Geometry: final body of the model. Coordinates: model frame, mm. A direction names the side the tool comes from. Give positions to 0.01 mm unless a question says otherwise; leave off trailing zeros. Order: outer loops, then holes, each group sorted by start corner. A loop starts at its lowest first (then second) coordinate and runs counter-clockwise, first axis right, second up. Notation, with made-up numbers: (10.5, -1.75) -> (61.5, -1.75) arc R12 cw to (61.5, 13.25) -> close; hole circle Ø3 at (55, 54.5). An arc over 180 degrees is marked (long way). One line per question, with ' | ' between items.
from build123d import *

# Parameters (mm, degrees)
SKETCH1_R           = 30
BOSS_EXTRUDE1_DEPTH = 4
BOSS_EXTRUDE2_START = -17
BOSS_EXTRUDE2_DEPTH = 17


with BuildPart() as part:
    # Sketch1 → Boss-Extrude1 (new body)
    with BuildSketch(Plane.XY):
        Circle(SKETCH1_R)
        with BuildLine():
            ThreePointArc((-12.727922061, -12.727922061), (0, -18), (12.727922061, -12.727922061))
            ThreePointArc((12.727922061, -12.727922061), (13.378240315, -9.458551421), (10.606601718, -7.606601718))
            ThreePointArc((10.606601718, -7.606601718), (9.458551421, -7.83496312), (8.485281374, -8.485281374))
            ThreePointArc((8.485281374, -8.485281374), (0, -12), (-8.485281374, -8.485281374))
            ThreePointArc((-8.485281374, -8.485281374), (-9.458551421, -7.83496312), (-10.606601718, -7.606601718))
            ThreePointArc((-10.606601718, -7.606601718), (-13.378240315, -9.458551421), (-12.727922061, -12.727922061))
        make_face(mode=Mode.SUBTRACT)
        with BuildLine():
            ThreePointArc((8.485281374, 8.485281374), (12.727922061, 8.485281374), (12.727922061, 12.727922061))
            ThreePointArc((12.727922061, 12.727922061), (6.888301783, 16.629831585), (0, 18))
            ThreePointArc((0, 18), (-6.888301783, 16.629831585), (-12.727922061, 12.727922061))
            ThreePointArc((-12.727922061, 12.727922061), (-12.727922061, 8.485281374), (-8.485281374, 8.485281374))
            ThreePointArc((-8.485281374, 8.485281374), (-4.592201188, 11.08655439), (0, 12))
            ThreePointArc((0, 12), (4.592201188, 11.08655439), (8.485281374, 8.485281374))
        make_face(mode=Mode.SUBTRACT)
        with BuildLine():
            ThreePointArc((0, -4.95), (-1.55, -6.5), (0, -8.05))
            ThreePointArc((0, -8.05), (1.55, -6.5), (0, -4.95))
        make_face(mode=Mode.SUBTRACT)
        with BuildLine():
            ThreePointArc((6, 1.55), (4.45, 0), (6, -1.55))
            ThreePointArc((6, -1.55), (7.55, 0), (6, 1.55))
        make_face(mode=Mode.SUBTRACT)
        with BuildLine():
            ThreePointArc((-6, 1.55), (-7.55, 0), (-6, -1.55))
            ThreePointArc((-6, -1.55), (-4.45, 0), (-6, 1.55))
        make_face(mode=Mode.SUBTRACT)
        with BuildLine():
            ThreePointArc((0, 4.95), (1.55, 6.5), (0, 8.05))
            ThreePointArc((0, 8.05), (-1.55, 6.5), (0, 4.95))
        make_face(mode=Mode.SUBTRACT)
        with BuildLine():
            ThreePointArc((0, 4.1), (-4.1, 0), (0, -4.1))
            ThreePointArc((0, -4.1), (4.1, 0), (0, 4.1))
        make_face(mode=Mode.SUBTRACT)
    extrude(amount=-BOSS_EXTRUDE1_DEPTH)

    # Sketch2 → Boss-Extrude2 (add)
    with BuildSketch(Plane(origin=(0, 0, -21), x_dir=(-1, 0, 0), z_dir=(0, 0, -1)).offset(BOSS_EXTRUDE2_START)):
        with BuildLine():
            ThreePointArc((0, -30), (30, 0), (0, 30))
            ThreePointArc((0, 30), (-30, 0), (0, -30))
        make_face()
        with BuildLine():
            ThreePointArc((0, 21), (-21, 0), (0, -21))
            ThreePointArc((0, -21), (21, 0), (0, 21))
        make_face(mode=Mode.SUBTRACT)
    extrude(amount=BOSS_EXTRUDE2_DEPTH)


solid = part.part
1) Set-up query: faces 1 (the flat face through (6, -6, 0)), 2 (the cylindrical face through (0, -12, -2)), 3 (the cylindrical face through (8.04, -19.4, -12.38)). Return all of +Z, -Z, +X, -X, +Y, -Y with unobstructed straight access to the full face (end or side cutting, diameter ignored); none if empty.
Check result:
face 1: +Z, +X, -X, +Y, -Y | face 2: +Z, -Z | face 3: -Z
2) Section C-C on x = 11.5. Return loops of the section in (y, z).
Check result:
outline: (-27.71, -21) -> (-17.57, -21) -> (-17.57, -4) -> (-13.85, -4) -> (-13.85, 0) -> (-27.71, 0) -> close; (-7.74, -4) -> (7.74, -4) -> (7.74, 0) -> (-7.74, 0) -> close; (13.85, -4) -> (17.57, -4) -> (17.57, -21) -> (27.71, -21) -> (27.71, 0) -> (13.85, 0) -> close
3) Pull-direction query (X, two-part tool) for faces 4 (the cylindrical face through (-12.77, 8.53, -1.97)), 5 (the flat face through (20.4, -6.2, -21)), 6 (the flat face through (-0.3, -4.4, -4)); classes: +X half, -X half, draft (parallel to the pull), parting line (faces both ways), or undercut.
Check result:
face 4: undercut | face 5: draft | face 6: undercut
4) Section B-B on y = 0. Return loops of the section in (x, z).
Check result:
outline: (-30, -21) -> (-21, -21) -> (-21, -4) -> (-7.55, -4) -> (-7.55, 0) -> (-30, 0) -> close; (-4.45, -4) -> (-4.1, -4) -> (-4.1, 0) -> (-4.45, 0) -> close; (4.1, -4) -> (4.45, -4) -> (4.45, 0) -> (4.1, 0) -> close; (7.55, -4) -> (21, -4) -> (21, -21) -> (30, -21) -> (30, 0) -> (7.55, 0) -> close
5) Section D-D on y = 15. Return loops of the section in (x, z), plus the area to 3 significant figures.
Check result:
outline: (-25.98, -21) -> (-14.7, -21) -> (-14.7, -4) -> (-9.95, -4) -> (-9.95, 0) -> (-25.98, 0) -> close; (9.95, -4) -> (14.7, -4) -> (14.7, -21) -> (25.98, -21) -> (25.98, 0) -> (9.95, 0) -> close | area: 512 mm^2
6) Section A-A on z = -1.75. Return loops of the section in (x, y).
Check result:
outline: circle Ø60 at (0, 0); hole (-12.73, -12.73) arc R18 ccw to (12.73, -12.73) arc R3 ccw to (8.49, -8.49) arc R12 cw to (-8.49, -8.49) arc R3 ccw to start; hole (-12.73, 12.73) arc R3 ccw to (-8.49, 8.49) arc R12 cw to (8.49, 8.49) arc R3 ccw to (12.73, 12.73) arc R18 ccw to start; hole circle Ø3.1 at (-6, 0); hole circle Ø8.2 at (0, 0); hole circle Ø3.1 at (0, -6.5); hole circle Ø3.1 at (0, 6.5); hole circle Ø3.1 at (6, 0)
7) Material intervals for probe 1 along X at (y, z) = (0, -1.25); probe 2 along X at (y, z) = (-11, -1.25); probe 3 along Y at (x, z) = (1, -1), sorted ascending. Write a range as from..to.
Check result:
probe 1: x = -30..-7.55, -4.45..-4.1, 4.1..4.45, 7.55..30 | probe 2: x = -27.91..-13.58, -4.8..4.8, 13.58..27.91 | probe 3: y = -29.98..-17.97, -11.96..-7.68, -5.32..-3.98, 3.98..5.32, 7.68..11.96, 17.97..29.98
8) Contact query for flat-ended pins moving along their axis: pin 1 Ø3 at (y, z) = (10.5, -4) entering from -X; pin 2 Ø25 at (x, y) = (0, 0) entering from -Z; pin 3 Ø12 at (x, z) = (11.5, -3) entering from -Y; pin 4 Ø1.9 at (x, y) = (0, -6.5) entering from +Z. Output: stop coordinate, or through.
Check result:
pin 1: stops at x = -28.62 | pin 2: stops at z = -4 | pin 3: stops at y = -29.49 | pin 4: passes through
